Here's how the part is built. I have some questions about the finished solid (model axes, mm). Round coordinates to 2 decimals unless told otherwise and drop trailing zeros. Write each loop counter-clockwise with the first axis right and the second up, starting at its lowest first coordinate (ties: lowest second). Pieces come first, ordered by that corner, then holes. Notation, with made-up numbers: (36.5, 58.5) -> (86.5, 58.5) arc R16 cw to (86.5, 76.5) -> close; hole circle Ø6 at (60.25, 38.25). An arc over 180 degrees is marked (long way). Put each result on its own line as item: value. Start each with the question number.
1. I need wall thicknesses on probe 1 along Y at (x, z) = (39, 0.1); probe 2 along Z at (x, y) = (15.5, 1.8); probe 3 along Y at (x, z) = (71.5, -2.1). Which ranges of each line are inside material? Lowest first, please. Write a range as from..to.
2. Suppose I cut it at A-A (y = 0.75). Please give me the cut outline in (x, z).
3. For pin 1 (1 mm diameter, centred on x = 31.5, z = -0.5, fed in from +Y), with a flat end and sliding along its axis, tell me the tip position at first contact or that it passes through.
4. Suppose I cut it at C-C (z = -1.6). Please give me the cut outline in (x, y), then the cut area to 3 significant figures.
5. Suppose I cut it at B-B (x = 84). Please give me the cut outline in (y, z), then the cut area to 3 significant figures.
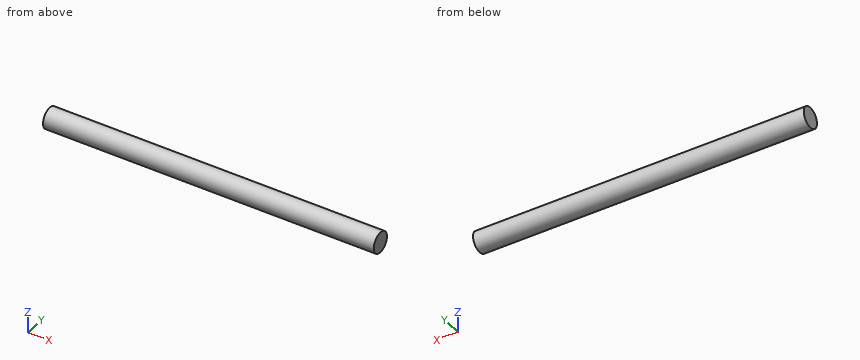
Autodesk Fusion 360 part; units mm, degrees
sketch "Sketch1" plane through (0, 0, 0) normal (0, 0, 1) x (1, 0, 0)
sketch "Sketch2" plane through (0, 0, 0) normal (1, 0, 0) x (0, 0, -1)
  circle A0 centre (0, 0) radius 2.5
  dimension "d1" = 5
extrude "Extrude1" add sketch "Sketch2" along normal blind 70
extrude "Extrude2" add 1 faces at (70, 0.2321, 0.8863) along direction (1, 0, 0) blind 20
extrude "Extrude3" cut 1 faces at (0, 0.2321, 0.8863) along direction (1, 0, 0) blind 10
extrude "Extrude4" cut 1 faces at (10, 0.2321, 0.8863) along direction (1, 0, 0) blind 10
extrude "Extrude5" add 1 faces at (20, 0.2321, 0.8863) along direction (-1, 0, 0) blind 10
Verdict:
1. probe 1: y = -2.5..2.5
1. probe 2: z = -1.73..1.73
1. probe 3: y = -1.36..1.36
2. outline: (10, -2.38) -> (90, -2.38) -> (90, 2.38) -> (10, 2.38) -> close
3. pin 1: stops at y = 2.5
4. outline: (10, -1.92) -> (90, -1.92) -> (90, 1.92) -> (10, 1.92) -> close
4. area: 307 mm^2
5. outline: circle Ø5 at (0, 0)
5. area: 19.6 mm^2
